The listing builds one solid part. Answer for the finished solid, in the listing's coordinates (mm). Round coordinates to 2 decimals unless told otherwise and drop trailing zeros. Loops run counter-clockwise (first coordinate to the right, second up) from the corner with the lowest first, then second, coordinate; pieces in that order, holes last. Notation, with made-up numbers: (0, 31) -> (5, 31) arc R23 ccw to (5, 46) -> close; hole circle Ø7 at (11.5, 86.25). An arc over 180 degrees is marked (long way). One line per question, with ' | ' between items.
from build123d import *

# Parameters (mm, degrees)
SKETCH_1_W          = 30
SKETCH_1_H          = 10
SKETCH_1_W_2        = 26
SKETCH_1_H_2        = 6
EXTRUDE_1_DEPTH     = 330
SKETCH_2_R          = 1.6
CUT_EXTRUDE_1_DEPTH = 331.492057393
SKETCH_3_R          = 1.6
SKETCH_3_R_2        = 1.65
CUT_EXTRUDE_2_DEPTH = 331.492057393
SKETCH_4_R          = 1.6
CUT_EXTRUDE_3_DEPTH = 332.398551596
SKETCH_6_W          = 28
SKETCH_6_H          = 8
CUT_EXTRUDE_5_DEPTH = 355
SKETCH_7_R          = 1.6
CUT_EXTRUDE_6_DEPTH = 14
SKETCH_9_W          = 30
SKETCH_9_H          = 10
CUT_EXTRUDE_7_DEPTH = 150


with BuildPart() as part:
    # 草图1 → 凸台-拉伸1 (new body)
    with BuildSketch(Plane.XY):
        Rectangle(SKETCH_1_W, SKETCH_1_H)
        Rectangle(SKETCH_1_W_2, SKETCH_1_H_2, mode=Mode.SUBTRACT)
    extrude(amount=EXTRUDE_1_DEPTH)

    # 草图2 → 切除-拉伸1 (cut, through all)
    with BuildSketch(Plane(origin=(0, 5, 0), x_dir=(1, 0, 0), z_dir=(0, 1, 0))):
        with Locations(Location((-11.3, -321, 0), (0, 0, 270))):
            Circle(SKETCH_2_R)
    extrude(amount=-CUT_EXTRUDE_1_DEPTH, mode=Mode.SUBTRACT)

    # 草图3 → 切除-拉伸2 (cut, through all)
    with BuildSketch(Plane(origin=(0, 5, 0), x_dir=(1, 0, 0), z_dir=(0, 1, 0))):
        with Locations(Location((5.907293091, -296.425438671, 0), (0, 0, 270))):
            Circle(SKETCH_3_R)
        with Locations(Location((0, -215, 0), (0, 0, 270))):
            Circle(SKETCH_3_R_2)
        with Locations(Location((0, -185, 0), (0, 0, 270))):
            Circle(SKETCH_3_R_2)
        with Locations(Location((0, -275, 0), (0, 0, 270))):
            Circle(SKETCH_3_R_2)
        with Locations(Location((0, -245, 0), (0, 0, 270))):
            Circle(SKETCH_3_R_2)
    extrude(amount=-CUT_EXTRUDE_2_DEPTH, mode=Mode.SUBTRACT)

    # 草图4 → 切除-拉伸3 (cut, through all)
    with BuildSketch(Plane.ZY.offset(15)):
        with Locations((170, 0)):
            Circle(SKETCH_4_R)
        with Locations((190, 0)):
            Circle(SKETCH_4_R)
        with Locations((210, 0)):
            Circle(SKETCH_4_R)
    extrude(amount=-CUT_EXTRUDE_3_DEPTH, mode=Mode.SUBTRACT)

    # 草图6 → 切除-拉伸5 (cut)
    with BuildSketch(Plane(origin=(0, 0, 0), x_dir=(-1, 0, 0), z_dir=(0, 0, -1))):
        Rectangle(SKETCH_6_W, SKETCH_6_H)
    extrude(amount=-CUT_EXTRUDE_5_DEPTH, mode=Mode.SUBTRACT)

    # 草图7 → 切除-拉伸6 (cut)
    with BuildSketch(Plane(origin=(0, 5, 0), x_dir=(1, 0, 0), z_dir=(0, 1, 0))):
        with Locations(Location((5.907293091, -321, 0), (0, 0, 270))):
            Circle(SKETCH_7_R)
        with Locations(Location((-11.3, -296.425438671, 0), (0, 0, 270))):
            Circle(SKETCH_7_R)
    extrude(amount=-CUT_EXTRUDE_6_DEPTH, mode=Mode.SUBTRACT)

    # 草图9 → 切除-拉伸7 (cut)
    with BuildSketch(Plane(origin=(0, 0, 0), x_dir=(-1, 0, 0), z_dir=(0, 0, -1))):
        Rectangle(SKETCH_9_W, SKETCH_9_H)
    extrude(amount=-CUT_EXTRUDE_7_DEPTH, mode=Mode.SUBTRACT)


solid = part.part
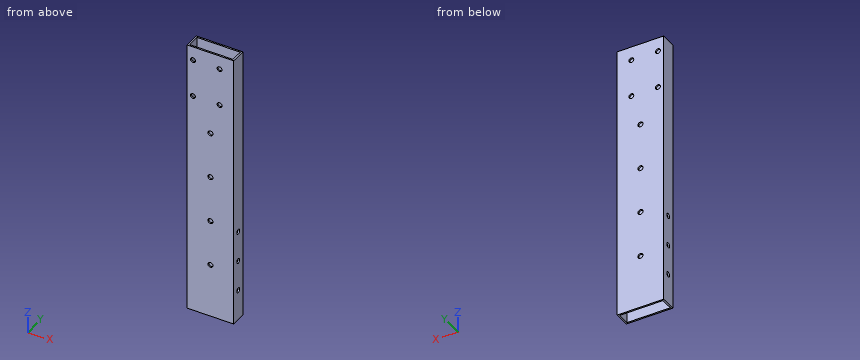
Q1. Find the intervals of material crossed by line 1 (X direction, y = -4.15, z = 321); line 2 (Y direction, x = -8.25, z = 266.5); line 3 (Y direction, x = -14.4, z = 190), in increasing order. Write a range as from..to.
Numbers:
line 1: -15..-12.9, -9.7..4.31, 7.51..15 | line 2: -5..-4, 4..5 | line 3: -5..-1.6, 1.6..5
Q2. A cutting plane is placed at A-A on z = 210. Give the vertices of the cut face in (x, y).
Numbers:
outline: (-15, -5) -> (15, -5) -> (15, -1.6) -> (14, -1.6) -> (14, -4) -> (-14, -4) -> (-14, -1.6) -> (-15, -1.6) -> close; (-15, 1.6) -> (-14, 1.6) -> (-14, 4) -> (14, 4) -> (14, 1.6) -> (15, 1.6) -> (15, 5) -> (-15, 5) -> close
Q3. A cutting plane is placed at D-D on z = 321. Give the vertices of the cut face in (x, y).
Numbers:
outline: (-15, -5) -> (-12.9, -5) -> (-12.9, -4) -> (-14, -4) -> (-14, 4) -> (-12.9, 4) -> (-12.9, 5) -> (-15, 5) -> close; (-9.7, -5) -> (4.31, -5) -> (4.31, -4) -> (-9.7, -4) -> close; (-9.7, 4) -> (4.31, 4) -> (4.31, 5) -> (-9.7, 5) -> close; (7.51, -5) -> (15, -5) -> (15, 5) -> (7.51, 5) -> (7.51, 4) -> (14, 4) -> (14, -4) -> (7.51, -4) -> close
Q4. A cutting plane is placed at B-B on x = -5.5. Give the vertices of the cut face in (y, z), plus the area to 3 significant figures.
Numbers:
outline: (-5, 150) -> (-4, 150) -> (-4, 330) -> (-5, 330) -> close; (4, 150) -> (5, 150) -> (5, 330) -> (4, 330) -> close | area: 360 mm^2
Q5. Given pin 1 Ø3.5 at (x, z) = (5.91, 296.43) entering from -Y, flat-ended and moving along its own axis, determine where the tip first touches the part or whether it passes through.
Numbers:
pin 1: y = -5
Q6. A cutting plane is placed at C-C on y = 0. Give the number of separate pieces and of enclosed holes in the cut face, plus the area to 3 significant figures.
Numbers:
separate pieces: 8 | enclosed holes: 0 | area: 341 mm^2
